Autodesk Inventor part; units mm, degrees
ref_plane "YZ Plane" through (0, 0, 0) normal (1, 0, 0) x (0, 1, 0)
ref_plane "XZ Plane" through (0, 0, 0) normal (0, 1, 0) x (-1, 0, 0)
ref_plane "XY Plane" through (0, 0, 0) normal (0, 0, 1) x (1, 0, 0)
sketch "Sketch1" plane through (0, 0, 0) normal (1, 0, 0) x (0, 1, 0)
  circle A0 centre (0, 0) radius 15.24
  circle A1 centre (9.779, 0) radius 1.7859
  circle A2 centre (0, -9.779) radius 1.7859
  circle A3 centre (-9.779, 0) radius 1.7859
  circle A4 centre (0, 9.779) radius 1.7859
  circle A5 centre (0, 0) radius 6.35
  arc A6 (-1.7785, -9.6159) -> (1.7785, -9.6159) centre (0, 0) ccw
  dimension "d0" = 30.48
  dimension "d2" = 3.5719
  dimension "d3" = 3.5719
  dimension "d4" = 3.5719
  dimension "d5" = 3.5719
  dimension "d6" = 12.7
extrude "Extrusion1" add sketch "Sketch1" along normal blind 5.08
sketch "Sketch5" plane through (5.08, 0, 0) normal (1, 0, 0) x (0, 0, -1)
  circle A0 centre (0, 0) radius 15.24
  arc A1 (0, -15.24) -> (0, 15.24) centre (0, 0) ccw
  line L0 (0, 15.24) -> (27.94, 15.24)
  line L1 (27.94, 15.24) -> (27.94, -15.24)
  line L2 (27.94, -15.24) -> (0, -15.24)
  dimension "d17" = 27.94
  dimension "d18" = 30.48
extrude "Extrusion3" add sketch "Sketch5" against normal blind 5.08 contours A0 L0 L1 L2
sketch "Sketch6" plane through (5.08, 0, 0) normal (1, 0, 0) x (0, 0, -1)
  line L0 (27.94, -15.24) -> (27.94, 15.24)
  line L1 (27.94, -15.24) -> (22.86, -15.24)
  line L2 (22.86, -15.24) -> (22.86, 15.6141)
  line L3 (22.86, 15.6141) -> (27.94, 15.6141)
  line L4 (27.94, 15.6141) -> (27.94, -15.24)
  point P0 (0, 0)
  dimension "d21" = 5.08
extrude "Extrusion4" add sketch "Sketch6" along normal blind 12.7
sketch "Sketch7" plane through (0, -15.24, -27.94) normal (0, 0, -1) x (-1, 0, 0)
  line L0 (-17.78, 30.8541) -> (-17.78, 0)
  line L1 (-17.78, 0) -> (-81.28, 0)
  line L2 (-81.28, 0) -> (-81.28, 101.6)
  line L3 (-81.28, 101.6) -> (-17.78, 101.6)
  line L4 (-17.78, 101.6) -> (-17.78, 0)
  line L5 (-5.08, 0) -> (-17.78, 0)
  line L6 (-17.78, 0) -> (-81.28, 0)
  line L7 (-81.28, 0) -> (-81.28, -12.7)
  line L8 (-81.28, -12.7) -> (-17.78, -12.7)
  line L9 (-17.78, -12.7) -> (-17.78, 0)
  point P0 (0, 15.24)
  dimension "d24" = 63.5
  dimension "d25" = 101.6
  dimension "d26" = 12.7
extrude "Extrusion5" add sketch "Sketch7" against normal blind 5.08
fillet "Fillet1" radius 3.175 11 edges at (5.08, 0, -22.86) (17.78, 86.36, -25.4) (81.28, 86.36, -25.4) (81.28, -27.94, -25.4) (0, 0, -27.94) (17.78, -27.94, -25.4) (49.53, -27.94, -22.86) (17.78, -21.59, -22.86) (17.78, 50.987, -22.86) (49.53, 86.36, -22.86) (81.28, 29.21, -22.86)
properties part number "GripperConstant"
The listing builds one solid part. Answer for the finished solid, in the listing's coordinates (mm). A direction names the side the tool comes from. Round coordinates to 2 decimals unless told otherwise and drop trailing zeros. Write each loop counter-clockwise with the first axis right and the second up, starting at its lowest first coordinate (ties: lowest second). Pieces come first, ordered by that corner, then holes. Notation, with made-up numbers: (1.5, 72) -> (8.5, 72) arc R26 cw to (8.5, 105) -> close; hole circle Ø5 at (-24, -15). An arc over 180 degrees is marked (long way). Answer as a JSON object with one key per item and string values. Group by question number.
Q1. Each of these flat-tipped pins is pushed along its axis until it touches: pin 1 Ø1.5 at (x, z) = (16, -26.5) entering from +Y; pin 2 Ø14.5 at (y, z) = (0, 0) entering from +X; pin 3 Ø1.5 at (y, z) = (-18, -27) entering from -X; pin 4 Ø5.5 at (y, z) = (-9.779, 0) entering from -X. Where does it stop, or does it pass through?
Q2. Determine the mould class of faces 1 (the face through (2.5, -1.38, 6.2)), 2 (the face through (18.7, -19.9, -23.8)), 3 (the face through (3, -15.24, -17)) for opening direction Y: pulls with the +Y half, pulls with the -Y half, needs draft (parallel to the pull), parting line crosses it, or undercut.
Q3. Which of the six approach directions +Z, -Z, +X, -X, +Y, -Y give full straight-line access (tool end or side, diameter ignored) to faces 4 (the face through (2.504, 7.995, -0.079)), 5 (the face through (18.7, 49.9, -23.8)), 6 (the face through (5.08, 3, -6))?
Q4. Section A-A (y = 0) is taken. Write down the section's boundary in (x, z) (3 decimals), plus the area to 3 significant figures.
Q5. Section B-B (x = 31.5) is taken. Write down the section's boundary in (y, z) (3 decimals).
Q6. Straight lines are drawn through the part: line 1 along Z through (x, y) = (3.95, 0); line 2 along Z through (x, y) = (1.2, 0); line 3 along Y through (x, z) = (5, -1.5). For each, find the intervals that lie inside material, in ascending order.
Q7. Section D-D (x = 9.5) is taken. Write down the section's boundary in (y, z), plus the area to 3 significant figures.
Q8. Section C-C (y = 79.5) is taken. Write down the section's boundary in (x, z) (3 decimals).
Check values:
{
 "1": {"pin 1": "y = 15.61", "pin 2": "x = 5.08", "pin 3": "x = 17.78", "pin 4": "x = 0"},
 "2": {"face 1": "undercut", "face 2": "needs draft", "face 3": "pulls with the -Y half"},
 "3": {"face 4": "+X, -X", "face 5": "+Z, -X, +Y", "face 6": "+Z, +X, +Y, -Y"},
 "4": {"outline": "(0, -24.765) arc R3.175 ccw to (3.175, -27.94) -> (81.28, -27.94) -> (81.28, -26.035) arc R3.175 ccw to (78.105, -22.86) -> (8.255, -22.86) arc R3.175 cw to (5.08, -19.685) -> (5.08, -11.565) -> (0, -11.565) -> close; (0, -7.993) -> (5.08, -7.993) -> (5.08, -6.35) -> (0, -6.35) -> close; (0, 6.35) -> (5.08, 6.35) -> (5.08, 7.993) -> (0, 7.993) -> close; (0, 11.565) -> (5.08, 11.565) -> (5.08, 15.24) -> (0, 15.24) -> close", "area": "503 mm^2"},
 "5": {"outline": "(-27.94, -27.94) -> (86.36, -27.94) -> (86.36, -26.035) arc R3.175 ccw to (83.185, -22.86) -> (-24.765, -22.86) arc R3.175 ccw to (-27.94, -26.035) -> close"},
 "6": {"line 1": "-27.94 to -11.56, -7.99 to -6.35, 6.35 to 7.99, 11.56 to 15.24", "line 2": "-27.25 to -11.56, -7.99 to -6.35, 6.35 to 7.99, 11.56 to 15.24", "line 3": "-15.24 to -10.75, -8.81 to -6.17, 6.17 to 8.81, 10.75 to 15.24"},
 "7": {"outline": "(-15.24, -27.94) -> (15.61, -27.94) -> (15.61, -22.86) -> (-15.24, -22.86) -> close", "area": "157 mm^2"},
 "8": {"outline": "(17.78, -27.94) -> (81.28, -27.94) -> (81.28, -26.035) arc R3.175 ccw to (78.105, -22.86) -> (20.955, -22.86) arc R3.175 ccw to (17.78, -26.035) -> close"}
}
